Job drawing, mm, ordinate dimensions from the low corner. One solid piece. Round coordinates to 2 decimals unless told otherwise and drop trailing zeros. Write each loop counter-clockwise with the first axis right and the second up, starting at its lowest first coordinate (ties: lowest second). Pieces come first, ordered by that corner, then holes. Notation, with made-up numbers: (52.5, 44.5) -> (102.5, 44.5) arc R12 cw to (102.5, 54.5) -> close; hole circle Ø2 at (34, 40.25). An arc over 180 degrees is marked (long way). Use CSV: the item, a comma, the result in double quotes. Start each with the question number.
(1) Probe line 1 (Y direction, x = 14.5, z = 0.7); line 2 (Y direction, x = 25, z = 0.4) (1 decimal); line 3 (X direction, y = 9, z = 0.8) (1 decimal). List the from-to ranges inside material, lowest first. Write a range as [from, to].
(2) Saw through at B-B (y = 9.25). Give the cut face in (x, z) (1 decimal).
(3) Saw through at C-C (z = 0.55). Count the separate pieces of the cut face and the enclosed holes in it, plus the area to 3 significant figures.
(4) Saw through at D-D (x = 5.75). Give the cut face in (y, z).
(5) Saw through at A-A (x = 13.5). Give the cut face in (y, z).
(6) Drop a flat-ended pin along its axis: pin 1 (10 mm diameter, centred on x = 15, y = 14.5, fed in from -Z). Give the stop position or say it passes through.
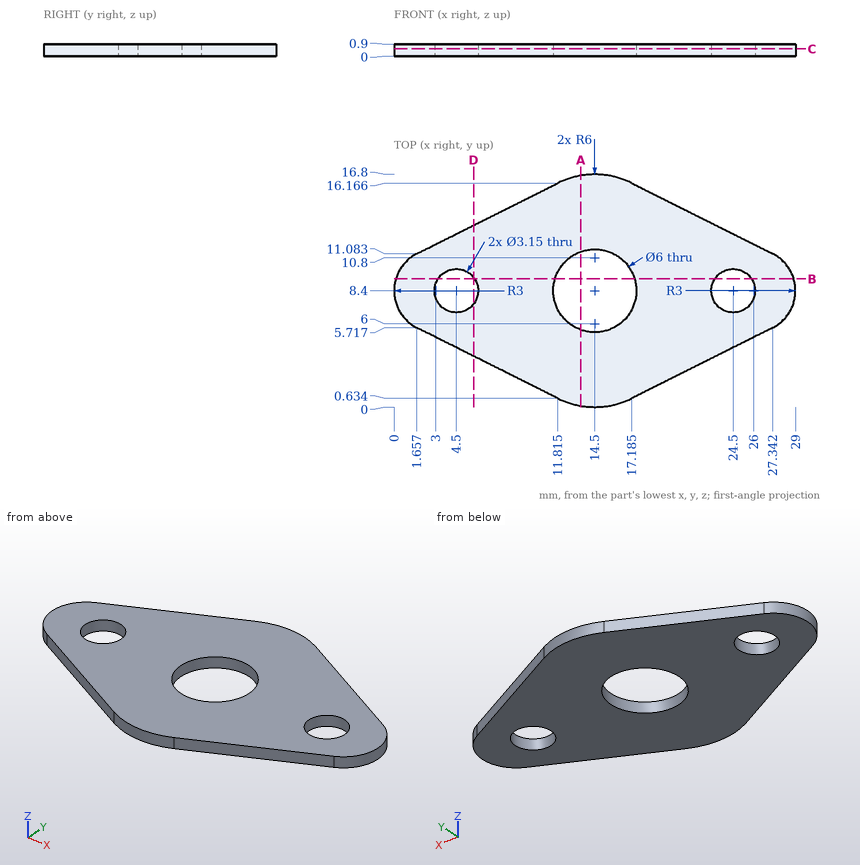
Answers:
1,line 1,"y = [0, 5.4], [11.4, 16.8]"
1,line 2,"y = [4.5, 6.9], [9.9, 12.3]"
1,line 3,"x = [0.1, 3], [6, 11.6], [17.4, 23], [26, 28.9]"
2,outline,"(0.1, 0) -> (3.2, 0) -> (3.2, 0.9) -> (0.1, 0.9) -> close; (5.8, 0) -> (11.6, 0) -> (11.6, 0.9) -> (5.8, 0.9) -> close; (17.4, 0) -> (23.2, 0) -> (23.2, 0.9) -> (17.4, 0.9) -> close; (25.8, 0) -> (28.9, 0) -> (28.9, 0.9) -> (25.8, 0.9) -> close"
3,separate pieces,"1"
3,enclosed holes,"3"
3,area,"269 mm²"
4,outline,"(3.67, 0) -> (7.44, 0) -> (7.44, 0.9) -> (3.67, 0.9) -> close; (9.36, 0) -> (13.13, 0) -> (13.13, 0.9) -> (9.36, 0.9) -> close"
5,outline,"(0.08, 0) -> (5.57, 0) -> (5.57, 0.9) -> (0.08, 0.9) -> close; (11.23, 0) -> (16.72, 0) -> (16.72, 0.9) -> (11.23, 0.9) -> close"
6,pin 1,"stops at z = 0"
